Part print with two shaded views. Sizes in mm from the minimum x, y, z corner. A direction names the side the tool comes from. Coordinates: 2 decimals unless noted, no trailing zeros. Order: outer loops, then holes, each group sorted by start corner. A loop starts at its lowest first (then second) coordinate and runs counter-clockwise, first axis right, second up. Notation, with made-up numbers: (18.25, 79) - (60.25, 79) arc R35 cw to (60.25, 118) - close; hole circle Ø1 at (-4.5, 33). An arc over 180 degrees is marked (long way). Return JSON: item names as keys, results as strings.
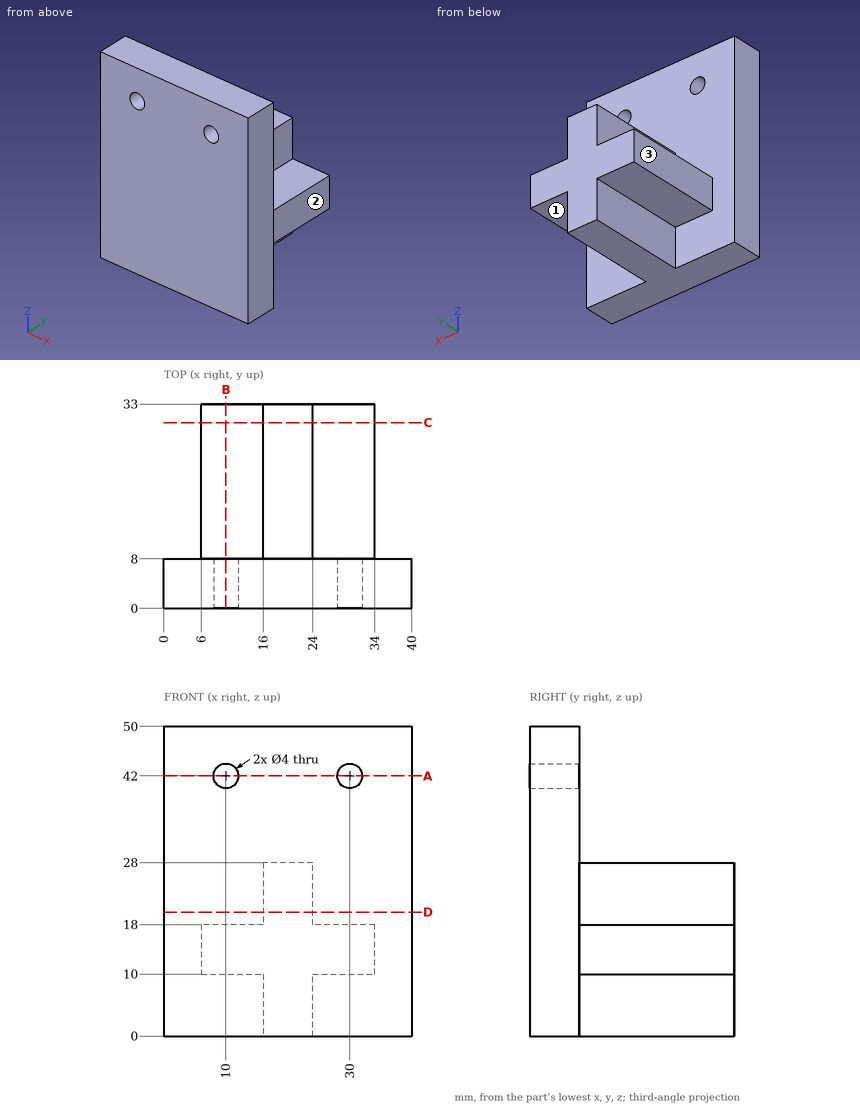
Item 1: Wall check: L1, parallel to X at y = 2.5, z = 42; L2, parallel to Y at x = 16, z = 47; L3, parallel to Z at x = 30, y = 6. Give the ranges that are in metal, low to high. Write a range as [from, to].
Findings below:
{"L1": "x = [0, 8], [12, 28], [32, 40]", "L2": "y = [0, 8]", "L3": "z = [0, 40], [44, 50]"}
Item 2: Drop flat-ended pins along their axis: P1, Ø11, axis at x = 9, y = 24, coming from the -Z side; P2, Ø3, axis at y = 14.5, z = 4.5, coming from the -X side; P3, Ø9, axis at x = 22, y = 16, coming from the +Z side; P4, Ø12, axis at x = 29, z = 25, coming from the -Y side. Give the stop position or say it passes through.
Findings below:
{"P1": "stops at z = 10", "P2": "stops at x = 16", "P3": "stops at z = 28", "P4": "stops at y = 0"}
Item 3: Band-saw the part on C-C, the plane y = 30. List the corners of the cut face in (x, z).
Findings below:
{"outline": "(6, 10) - (16, 10) - (16, 0) - (24, 0) - (24, 10) - (34, 10) - (34, 18) - (24, 18) - (24, 28) - (16, 28) - (16, 18) - (6, 18) - close"}
Item 4: Band-saw the part on B-B, the plane x = 10. List the corners of the cut face in (y, z).
Findings below:
{"outline": "(0, 0) - (8, 0) - (8, 10) - (33, 10) - (33, 18) - (8, 18) - (8, 40) - (0, 40) - close; (0, 44) - (8, 44) - (8, 50) - (0, 50) - close"}
Item 5: Band-saw the part on D-D, the plane z = 20. List the corners of the cut face in (x, y).
Findings below:
{"outline": "(0, 0) - (40, 0) - (40, 8) - (24, 8) - (24, 33) - (16, 33) - (16, 8) - (0, 8) - close"}
Item 6: Which spindle directions (+Z, -Z, +X, -X, +Y, -Y) get a long thin tool onto all of the face, cutting with end or side? Do the marked faces 1, 2 and 3. Say none if no direction does.
Findings below:
{"face 1": "-Z, +X, +Y", "face 2": "+Z, -Z, +X, +Y", "face 3": "+Z, -Z, -X, +Y"}
Item 7: Band-saw the part on A-A, the plane z = 42. List the corners of the cut face in (x, y), then the cut area to 3 significant figures.
Findings below:
{"outline": "(0, 0) - (8, 0) - (8, 8) - (0, 8) - close; (12, 0) - (28, 0) - (28, 8) - (12, 8) - close; (32, 0) - (40, 0) - (40, 8) - (32, 8) - close", "area": "256 mm²"}
